Check sheet for the modelled part. Datum: model origin and axes. Units: mm. Coordinates: 2 decimals unless noted, no trailing zeros. Write each loop counter-clockwise with the first axis right and the second up, starting at its lowest first coordinate (ties: lowest second). Pieces come first, ordered by that corner, then holes. Notation, with made-up numbers: (58.25, 55) -> (101.25, 55) arc R23 cw to (101.25, 90) -> close; hole circle Ø3 at (10.25, -22.75). An arc over 180 degrees is marked (long way). Put each result on its own line as item: value.
```python
from build123d import *

# Parameters (mm, degrees)
SKETCH3_R           = 100
BOSS_EXTRUDE1_DEPTH = 3
SKETCH4_R           = 5
BOSS_EXTRUDE2_DEPTH = 20
SKETCH5_R           = 2
BOSS_EXTRUDE3_DEPTH = 10


with BuildPart() as part:
    # Sketch3 → Boss-Extrude1 (new body)
    with BuildSketch(Plane(origin=(0, 0, 0), x_dir=(1, 0, 0), z_dir=(0, 1, 0))):
        with Locations(Location((0, 0, 0), (0, 0, 270))):
            Circle(SKETCH3_R)
    extrude(amount=BOSS_EXTRUDE1_DEPTH)

    # Sketch4 → Boss-Extrude2 (add)
    with BuildSketch(Plane(origin=(0, 3, 0), x_dir=(1, 0, 0), z_dir=(0, 1, 0))):
        with Locations(Location((-50, 50, 0), (0, 0, 270))):
            Circle(SKETCH4_R)
        with Locations(Location((50, 50, 0), (0, 0, 270))):
            Circle(SKETCH4_R)
        with Locations(Location((50, -50, 0), (0, 0, 270))):
            Circle(SKETCH4_R)
        with Locations(Location((-50, -50, 0), (0, 0, 270))):
            Circle(SKETCH4_R)
    extrude(amount=BOSS_EXTRUDE2_DEPTH)

    # Sketch5 → Boss-Extrude3 (add)
    with BuildSketch(Plane(origin=(0, 23, 0), x_dir=(1, 0, 0), z_dir=(0, 1, 0))):
        with Locations(Location((50, -50, 0), (0, 0, 270))):
            Circle(SKETCH5_R)
        with Locations(Location((-50, -50, 0), (0, 0, 270))):
            Circle(SKETCH5_R)
        with Locations(Location((-50, 50, 0), (0, 0, 270))):
            Circle(SKETCH5_R)
        with Locations(Location((50, 50, 0), (0, 0, 270))):
            Circle(SKETCH5_R)
    extrude(amount=BOSS_EXTRUDE3_DEPTH)


solid = part.part
```
Q1. Depth check by flat-ended pin: P1, Ø8, axis at x = 48, z = 50.5, coming from the +Y side; P2, Ø8, axis at x = -44, y = 16.5, coming from the +Z side; P3, Ø10, axis at x = -56, y = 12, coming from the +Z side; P4, Ø2, axis at x = -60.5, z = 29, coming from the +Y side. Enter the tip coordinate at first touch or a pass-through.
Recorded:
P1: stops at y = 33
P2: stops at z = 54.58
P3: stops at z = 54.9
P4: stops at y = 3
Q2. Cross-section at A-A (y = 30.5). Record the cut outline in (x, z).
Recorded:
outline: circle Ø4 at (-50, -50); circle Ø4 at (-50, 50); circle Ø4 at (50, -50); circle Ø4 at (50, 50)
Q3. Cross-section at C-C (z = -27). Record the cut outline in (x, y).
Recorded:
outline: (-96.29, 0) -> (96.29, 0) -> (96.29, 3) -> (-96.29, 3) -> close
Q4. Cross-section at B-B (x = 0). Record the cut outline in (y, z).
Recorded:
outline: (0, -100) -> (3, -100) -> (3, 100) -> (0, 100) -> close
Q5. Mould release check, pull along X, two halves, no side actions. Record for faces 1 (the cylindrical face through (30.04, 1.48, 95.38)), 2 (the flat face through (1, 0, -1)), 3 (the cylindrical face through (54.957, 12.86, 49.349)), 4 (the cylindrical face through (54.957, 12.86, -50.651)): released by +X, released by -X, zero draft, split by the parting line, or undercut.
Recorded:
face 1: split by the parting line
face 2: zero draft
face 3: undercut
face 4: undercut
Q6. Material ranges on line 1 along Y through (x, z) = (-84, -40.5); line 2 along X through (y, z) = (9.5, 54); line 3 along Z through (x, y) = (49, 3.5), recorded low to high.
Recorded:
line 1: y = 0 to 3
line 2: x = -53 to -47, 47 to 53
line 3: z = -54.9 to -45.1, 45.1 to 54.9
Q7. Cross-section at D-D (y = 6). Record the cut outline in (x, z), plus the area to 3 significant figures.
Recorded:
outline: circle Ø10 at (-50, -50); circle Ø10 at (-50, 50); circle Ø10 at (50, -50); circle Ø10 at (50, 50)
area: 314 mm2
